Could you check a few things on this model? Use its own coordinates, in mm. A direction names the side the tool comes from. Coordinates: 2 decimals unless noted, no trailing zeros. Order: outer loops, then holes, each group sorted by start corner. A loop starts at its lowest first (then second) coordinate and runs counter-clockwise, first axis right, second up. Notation, with made-up numbers: (73, 81) - (87, 81) arc R29 ccw to (87, 116) - close; hole circle Ø10 at (25, 76.25). An arc over 180 degrees is marked (long way). One line per item, written item: value.
from build123d import *

# Parameters (mm, degrees)
SKETCH1_R           = 135
BOSS_EXTRUDE1_DEPTH = 20
SKETCH3_R           = 142.5
BOSS_EXTRUDE3_DEPTH = 10
SKETCH4_W           = 25
SKETCH4_H           = 70
BOSS_EXTRUDE4_DEPTH = 80
CUT_EXTRUDE1_START  = -130
CUT_EXTRUDE1_DEPTH  = 130
SKETCH6_R           = 10
CUT_EXTRUDE2_DEPTH  = 273.740719365


# Read off the part's stored shape, not the designer's step: Cut-Extrude1
with BuildPart() as part:
    # Sketch1 → Boss-Extrude1 (new body)
    with BuildSketch(Plane(origin=(0, 0, 0), x_dir=(1, 0, 0), z_dir=(0, 1, 0))):
        with Locations(Location((0, 0, 0), (0, 0, 270))):
            Circle(SKETCH1_R)
    extrude(amount=BOSS_EXTRUDE1_DEPTH)

    # Sketch3 → Boss-Extrude3 (add)
    with BuildSketch(Plane(origin=(0, 20, 0), x_dir=(1, 0, 0), z_dir=(0, 1, 0))):
        with Locations(Location((0, 0, 0), (0, 0, 270))):
            Circle(SKETCH3_R)
    extrude(amount=BOSS_EXTRUDE3_DEPTH)

    # Sketch4 → Boss-Extrude4 (add)
    with BuildSketch(Plane(origin=(0, 30, 0), x_dir=(1, 0, 0), z_dir=(0, 1, 0))):
        with Locations((-52.5, 0)):
            Rectangle(SKETCH4_W, SKETCH4_H)
        with Locations((52.5, 0)):
            Rectangle(SKETCH4_W, SKETCH4_H)
    extrude(amount=BOSS_EXTRUDE4_DEPTH)

    # Cut-Extrude1 outline → Cut-Extrude1 (cut)
    with BuildSketch(Plane(origin=(65, 0, 0), x_dir=(0, 0, -1), z_dir=(1, 0, 0)).offset(CUT_EXTRUDE1_START)):
        with BuildLine():
            ThreePointArc((-35, 70), (0, 105), (35, 70))
            Line((35, 70), (35, 110))
            Line((35, 110), (-35, 110))
            Line((-35, 110), (-35, 70))
        make_face()
    extrude(amount=CUT_EXTRUDE1_DEPTH, mode=Mode.SUBTRACT)

    # Sketch6 → Cut-Extrude2 (cut, through all)
    with BuildSketch(Plane(origin=(65, 0, 0), x_dir=(0, 0, -1), z_dir=(1, 0, 0))):
        with Locations((0, 70)):
            Circle(SKETCH6_R)
    extrude(amount=-CUT_EXTRUDE2_DEPTH, mode=Mode.SUBTRACT)


solid = part.part
Item 1: I want a section at C-C on y = 65. Please give me the cut outline in (x, z), then the cut area to 3 significant figures.
Conclusion:
outline: (-65, -35) - (-40, -35) - (-40, -8.66) - (-65, -8.66) - close; (-65, 8.66) - (-40, 8.66) - (-40, 35) - (-65, 35) - close; (40, -35) - (65, -35) - (65, -8.66) - (40, -8.66) - close; (40, 8.66) - (65, 8.66) - (65, 35) - (40, 35) - close
area: 2,630 mm²
Item 2: If I drill on probe 1 along Y at (x, z) = (-49, 0); probe 2 along X at (y, z) = (64, -10.5); probe 3 along Y at (x, z) = (65.5, 103), over which ranges is the centre line in solid material (lowest first)?
Conclusion:
probe 1: 0 to 60, 80 to 105
probe 2: -65 to -40, 40 to 65
probe 3: 0 to 30
Item 3: I want a section at D-D on x = -31. Please give me the cut outline in (y, z), then the cut area to 3 significant figures.
Conclusion:
outline: (0, -131.39) - (20, -131.39) - (20, -139.09) - (30, -139.09) - (30, 139.09) - (20, 139.09) - (20, 131.39) - (0, 131.39) - close
area: 8,040 mm²
Item 4: For faces 1 (the face through (-53, 50, 35)), 2 (the face through (-65, 59, 0)), 3 (the face through (52, 50, -35)), 4 (the face through (-119.77, 9.86, 62.29)), which set-ups out of +Z, -Z, +X, -X, +Y, -Y let a thin tool reach every point of the face, with its end or its side?
Conclusion:
face 1: +Z, +X, -X, +Y
face 2: +Z, -Z, -X, +Y
face 3: -Z, +X, -X, +Y
face 4: -Y
Item 5: I want a section at B-B on y = 35.5. Please give me the cut outline in (x, z), then the cut area to 3 significant figures.
Conclusion:
outline: (-65, -35) - (-40, -35) - (-40, 35) - (-65, 35) - close; (40, -35) - (65, -35) - (65, 35) - (40, 35) - close
area: 3,500 mm²
Item 6: I'm going to push flat-ended pins straight in: pin 1 Ø1.5 at (y, z) = (72, 10.5) entering from +X; pin 2 Ø12 at (y, z) = (70, 0) entering from -X; pin 3 Ø12 at (y, z) = (29, 76.5) entering from -X; pin 4 Ø5 at (x, y) = (-34.5, 25) entering from +Z. Where does each tip first touch, or does it pass through?
Conclusion:
pin 1: x = 65
pin 2: through
pin 3: x = -123.84
pin 4: z = 138.86
Item 7: I want a section at A-A on z = 0. Please give me the cut outline in (x, y).
Conclusion:
outline: (-142.5, 20) - (-135, 20) - (-135, 0) - (135, 0) - (135, 20) - (142.5, 20) - (142.5, 30) - (65, 30) - (65, 60) - (40, 60) - (40, 30) - (-40, 30) - (-40, 60) - (-65, 60) - (-65, 30) - (-142.5, 30) - close; (-65, 80) - (-40, 80) - (-40, 105) - (-65, 105) - close; (40, 80) - (65, 80) - (65, 105) - (40, 105) - close
Item 8: Thinking about a two-plate mould opening in X: for faces 5 (the face through (65, 59, 0)), 6 (the face through (-53, 50, -35)), 7 (the face through (40, 59, 0)), which applies, pulls with the +X half, pulls with the -X half, needs draft (parallel to the pull), parting line crosses it, or undercut?
Conclusion:
face 5: pulls with the +X half
face 6: needs draft
face 7: undercut
